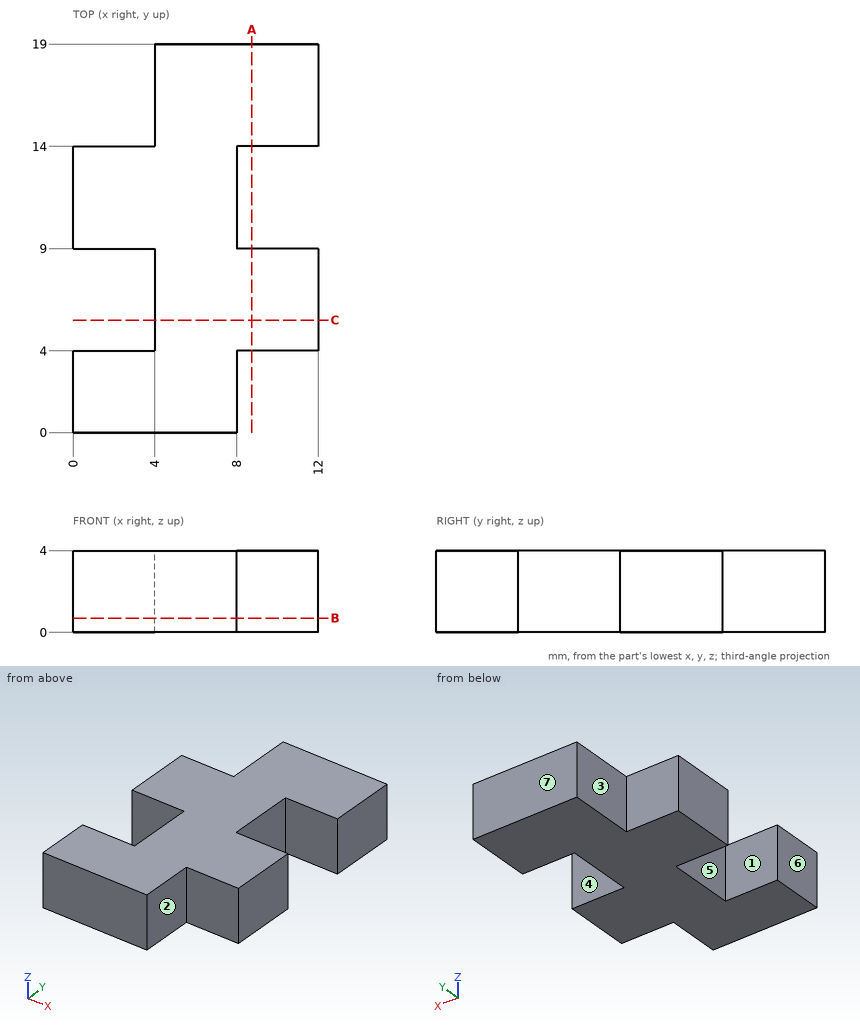
Answer from the drawing. Dimensions are ordinates in mm from the lowest x, y and z of the part. A direction names the side the tool comes from. Round coordinates to 2 decimals unless told otherwise and drop trailing zeros. Order: outer loops, then holes, each group sorted by start corner. A loop starts at its lowest first (then second) coordinate and runs counter-clockwise, first axis right, second up.
1) The mould has two halves that part along Y. Classify the marked faces 5, 6 and 7: released by +Y, released by -Y, zero draft, split by the parting line, or undercut.
2) Straight lines are drawn through the part: L1, parallel to Y at x = 1, z = 1.7; L2, parallel to Y at x = 9.25, z = 2.45; L3, parallel to X at y = 1.75, z = 3.4. For each, find the intervals that lie inside material, in ascending order.
3) The part is cut by section A-A on x = 8.75. Write down the section's boundary in (y, z), plus the area to 3 significant figures.
4) The part is cut by section B-B on z = 0.7. Write down the section's boundary in (x, y), plus the area to 3 significant figures.
5) The part is cut by section C-C on y = 5.5. Write down the section's boundary in (x, z).
6) Flat-ended cylindrical pins translate along their axes: pin 1 (1.5 mm diameter, centred on x = 10, y = 8, fed in from -Z); pin 2 (1.2 mm diameter, centred on x = 3, z = 2.5, fed in from +Y); pin 3 (1.2 mm diameter, centred on x = 9, z = 2.5, fed in from -Y). Find the tip coordinate at first contact, or state that the pin passes through.
7) For the marked faces 1, 2, 3 and 4, determine the directions among +Z, -Z, +X, -X, +Y, -Y from which every point of the face is accessible in a straight line to the end or side of a thin tool.
Resolved:
1. face 5: undercut
1. face 6: zero draft
1. face 7: released by +Y
2. L1: y = 0 to 4, 9 to 14
2. L2: y = 4 to 9, 14 to 19
2. L3: x = 0 to 8
3. outline: (4, 0) - (9, 0) - (9, 4) - (4, 4) - close; (14, 0) - (19, 0) - (19, 4) - (14, 4) - close
3. area: 40.0 mm2
4. outline: (0, 0) - (8, 0) - (8, 4) - (12, 4) - (12, 9) - (8, 9) - (8, 14) - (12, 14) - (12, 19) - (4, 19) - (4, 14) - (0, 14) - (0, 9) - (4, 9) - (4, 4) - (0, 4) - close
4. area: 152 mm2
5. outline: (4, 0) - (12, 0) - (12, 4) - (4, 4) - close
6. pin 1: stops at z = 0
6. pin 2: stops at y = 14
6. pin 3: stops at y = 4
7. face 1: +Z, -Z, -X
7. face 2: +Z, -Z, +X, -Y
7. face 3: +Z, -Z, -X, +Y
7. face 4: +Z, -Z, +X
